Verification items for the finished model (mm, model axes). A direction names the side the tool comes from. Round coordinates to 2 decimals unless told otherwise and drop trailing zeros. Order: outer loops, then holes, each group sorted by start corner. A loop starts at its lowest first (then second) coordinate and runs counter-clockwise, first axis right, second up. Notation, with made-up numbers: (55, 10) -> (114, 10) arc R27 cw to (114, 29) -> close; hole circle Ø9 at (-27.75, -23). An arc over 180 degrees is marked (long way). Put each result on its own line as item: value.
from build123d import *
from build123d.topology import SkipClean

# Parameters (mm, degrees)
SKETCH1_R           = 21.082
SKETCH1_R_2         = 17.526
BOSS_EXTRUDE1_DEPTH = 254
BOSS_EXTRUDE2_START = 6.35
SKETCH2_R           = 21.082
BOSS_EXTRUDE2_DEPTH = 6.35
SKETCH3_R           = 25.868376463
CUT_EXTRUDE1_DEPTH  = 127
SKETCH4_R           = 34.925
SKETCH4_R_2         = 19.091061219
BOSS_EXTRUDE3_DEPTH = 3.175
CUT_EXTRUDE2_DEPTH  = 143.203142546
CIRPATTERN1_COUNT   = 12
SKETCH6_R           = 21.082
CUT_EXTRUDE3_DEPTH  = 6.35
SKETCH7_R           = 21.082
BOSS_EXTRUDE4_DEPTH = 6.35
CUT_EXTRUDE5_DEPTH  = 137.26632471
BOSS_EXTRUDE5_DEPTH = 3.175
SKETCH13_R          = 20.701
SKETCH13_R_2        = 18.0848
CUT_EXTRUDE6_DEPTH  = 1.016
SKETCH14_R          = 22.3012
SKETCH14_R_2        = 20.701
BOSS_EXTRUDE6_DEPTH = 3.175
SKETCH15_R          = 3.175
SKETCH15_R_2        = 21.082
BOSS_EXTRUDE7_DEPTH = 123.825
SKETCH17_R          = 47.464750001
SKETCH17_R_2        = 22.3012
CUT_EXTRUDE7_DEPTH  = 120.65
SKETCH18_R          = 17.526
CUT_EXTRUDE8_DEPTH  = 134.883658048
CUT_EXTRUDE9_START  = -1.016
SKETCH19_R          = 20.701
SKETCH19_R_2        = 18.0848
CUT_EXTRUDE9_DEPTH  = 1.016
SKETCH20_R          = 43.35542212
CUT_EXTRUDE10_DEPTH = 25.4
SKETCH21_R          = 25.927665562
CUT_EXTRUDE11_DEPTH = 38.1
SKETCH22_R          = 20.063036937
BOSS_EXTRUDE8_DEPTH = 3.175


with BuildPart() as part:
    # Sketch1 → Boss-Extrude1 (new body)
    with BuildSketch(Plane.XY):
        Circle(SKETCH1_R)
        Circle(SKETCH1_R_2, mode=Mode.SUBTRACT)
    extrude(amount=BOSS_EXTRUDE1_DEPTH)

    # Sketch2 → Boss-Extrude2 (add)
    with BuildSketch(Plane(origin=(0, 0, 0), x_dir=(-1, 0, 0), z_dir=(0, 0, -1)).offset(BOSS_EXTRUDE2_START)):
        Circle(SKETCH2_R)
    extrude(amount=-BOSS_EXTRUDE2_DEPTH)

    # Sketch3 → Cut-Extrude1 (cut)
    with BuildSketch(Plane.XY.offset(254)):
        Circle(SKETCH3_R)
    extrude(amount=-CUT_EXTRUDE1_DEPTH, mode=Mode.SUBTRACT)

    # Sketch4 → Boss-Extrude3 (add)
    with BuildSketch(Plane.XY.offset(127)):
        Circle(SKETCH4_R)
        Circle(SKETCH4_R_2, mode=Mode.SUBTRACT)
    extrude(amount=-BOSS_EXTRUDE3_DEPTH)

    # Sketch5 → Cut-Extrude2 (cut, through all)
    with BuildSketch(Plane.XY.offset(127)):
        with BuildLine():
            ThreePointArc((0, 31.75), (-3.175, 28.575), (0, 25.4))
            Line((0, 25.4), (0, 31.75))
        make_face()
        with BuildLine():
            Line((0, 31.75), (0, 25.4))
            ThreePointArc((0, 25.4), (2.24506403, 26.32993597), (3.175, 28.575))
            ThreePointArc((3.175, 28.575), (2.24506403, 30.82006403), (0, 31.75))
        make_face()
    cut_extrude2 = extrude(amount=-CUT_EXTRUDE2_DEPTH, mode=Mode.SUBTRACT)

    # CirPattern1: Cut-Extrude2 ×12 about axis
    cirpattern1_axis = Axis((0, 0, 0), (0, 0, 1))
    for i in range(1, CIRPATTERN1_COUNT):
        add(cut_extrude2.rotate(cirpattern1_axis, i * 360 / CIRPATTERN1_COUNT), mode=Mode.SUBTRACT)

    # Sketch6 → Cut-Extrude3 (cut)
    with BuildSketch(Plane(origin=(0, 0, -6.35), x_dir=(-1, 0, 0), z_dir=(0, 0, -1))):
        Circle(SKETCH6_R)
    extrude(amount=-CUT_EXTRUDE3_DEPTH, mode=Mode.SUBTRACT)

    # Sketch7 → Boss-Extrude4 (add)
    with BuildSketch(Plane(origin=(0, 0, 0), x_dir=(-1, 0, 0), z_dir=(0, 0, -1))):
        Circle(SKETCH7_R)
    extrude(amount=-BOSS_EXTRUDE4_DEPTH)

    # Sketch8 → Cut-Extrude5 (cut, through all)
    with BuildSketch(Plane.XY.offset(127)):
        with BuildLine():
            ThreePointArc((18.828599641, 18.828599641), (22.949516837, 21.527350272), (27.854121372, 21.069018667))
            ThreePointArc((27.854121372, 21.069018667), (0, 34.925), (-27.854121372, 21.069018667))
            ThreePointArc((-27.854121372, 21.069018667), (-22.949516837, 21.527350272), (-18.828599641, 18.828599641))
            Line((-18.828599641, 18.828599641), (-14.907225161, 14.907225161))
            ThreePointArc((-14.907225161, 14.907225161), (0, 21.082), (14.907225161, 14.907225161))
            Line((14.907225161, 14.907225161), (18.828599641, 18.828599641))
        make_face()
        with BuildLine():
            ThreePointArc((14.907225161, -14.907225161), (0, -21.082), (-14.907225161, -14.907225161))
            Line((-14.907225161, -14.907225161), (-18.828599641, -18.828599641))
            ThreePointArc((-18.828599641, -18.828599641), (-22.949516837, -21.527350272), (-27.854121372, -21.069018667))
            ThreePointArc((-27.854121372, -21.069018667), (0, -34.925), (27.854121372, -21.069018667))
            ThreePointArc((27.854121372, -21.069018667), (22.949516837, -21.527350272), (18.828599641, -18.828599641))
            Line((18.828599641, -18.828599641), (14.907225161, -14.907225161))
        make_face()
    extrude(amount=-CUT_EXTRUDE5_DEPTH, mode=Mode.SUBTRACT)

    # Sketch11 → Boss-Extrude5 (add)
    with BuildSketch(Plane.XY.offset(127)):
        with BuildLine():
            ThreePointArc((31.206854634, 18.017286001), (29.767943301, 19.804028486), (27.854121372, 21.069018667))
            ThreePointArc((27.854121372, 21.069018667), (34.925, 0), (27.854121372, -21.069018667))
            ThreePointArc((27.854121372, -21.069018667), (29.767943301, -19.804028486), (31.206854634, -18.017286001))
            ThreePointArc((31.206854634, -18.017286001), (36.034571885, 0), (31.206854634, 18.017286001))
        make_face()
        with BuildLine():
            ThreePointArc((-27.854121372, 21.069018667), (-29.767943301, 19.804028486), (-31.206854634, 18.017286001))
            ThreePointArc((-31.206854634, 18.017286001), (-36.034571885, -1.77e-07), (-31.206854456, -18.017286308))
            ThreePointArc((-31.206854456, -18.017286308), (-29.767943169, -19.804028605), (-27.854121372, -21.069018667))
            ThreePointArc((-27.854121372, -21.069018667), (-34.925, 0), (-27.854121372, 21.069018667))
        make_face()
    extrude(amount=-BOSS_EXTRUDE5_DEPTH)

    # Sketch13 → Cut-Extrude6 (cut)
    with BuildSketch(Plane.XY.offset(127)):
        Circle(SKETCH13_R)
        Circle(SKETCH13_R_2, mode=Mode.SUBTRACT)
    extrude(amount=-CUT_EXTRUDE6_DEPTH, mode=Mode.SUBTRACT)

    # Sketch14 → Boss-Extrude6 (add)
    with BuildSketch(Plane.XY.offset(127)):
        Circle(SKETCH14_R)
        Circle(SKETCH14_R_2, mode=Mode.SUBTRACT)
    extrude(amount=-BOSS_EXTRUDE6_DEPTH)

    # Sketch15 → Boss-Extrude7 (add)
    with BuildSketch(Plane(origin=(0, 0, 123.825), x_dir=(-1, 0, 0), z_dir=(0, 0, -1))):
        with BuildLine():
            ThreePointArc((31.206854667, 18.017285943), (25.234555257, 21.731100369), (18.828599641, 18.828599641))
            Line((18.828599641, 18.828599641), (15.769329749, 15.769329749))
            ThreePointArc((15.769329749, 15.769329749), (0, 22.3012), (-15.769329749, 15.769329749))
            Line((-15.769329749, 15.769329749), (-18.828599641, 18.828599641))
            ThreePointArc((-18.828599641, 18.828599641), (-25.234555257, 21.731100369), (-31.206854667, 18.017285943))
            ThreePointArc((-31.206854667, 18.017285943), (-36.034571885, 0), (-31.206854667, -18.017285943))
            ThreePointArc((-31.206854667, -18.017285943), (-25.234555257, -21.731100369), (-18.828599641, -18.828599641))
            Line((-18.828599641, -18.828599641), (-15.769329749, -15.769329749))
            ThreePointArc((-15.769329749, -15.769329749), (0, -22.3012), (15.769329749, -15.769329749))
            Line((15.769329749, -15.769329749), (18.828599641, -18.828599641))
            ThreePointArc((18.828599641, -18.828599641), (25.234555257, -21.731100369), (31.206854667, -18.017285943))
            ThreePointArc((31.206854667, -18.017285943), (36.034571885, 0), (31.206854667, 18.017285943))
        make_face()
        with Locations(Location((28.575, 0, 0), (0, 0, 90))):
            Circle(SKETCH15_R, mode=Mode.SUBTRACT)
        with Locations(Location((-24.746675913, -14.2875, 0), (0, 0, 300))):
            Circle(SKETCH15_R, mode=Mode.SUBTRACT)
        with Locations(Location((-24.746675913, 14.2875, 0), (0, 0, 240))):
            Circle(SKETCH15_R, mode=Mode.SUBTRACT)
        with Locations(Location((-28.575, 0, 0), (0, 0, 270))):
            Circle(SKETCH15_R, mode=Mode.SUBTRACT)
        Circle(SKETCH15_R_2, mode=Mode.SUBTRACT)
        with Locations(Location((24.746675913, -14.2875, 0), (0, 0, 60))):
            Circle(SKETCH15_R, mode=Mode.SUBTRACT)
        with Locations(Location((24.746675913, 14.2875, 0), (0, 0, 120))):
            Circle(SKETCH15_R, mode=Mode.SUBTRACT)
    extrude(amount=BOSS_EXTRUDE7_DEPTH)

    # Sketch17 → Cut-Extrude7 (cut)
    with BuildSketch(Plane.XY.offset(123.825)):
        Circle(SKETCH17_R)
        with Locations(Location((0, 0, 0), (0, 0, 315))):
            Circle(SKETCH17_R_2, mode=Mode.SUBTRACT)
    extrude(amount=-CUT_EXTRUDE7_DEPTH, mode=Mode.SUBTRACT)

    # Sketch18 → Cut-Extrude8 (cut, through all)
    with BuildSketch(Plane.XY.offset(127)):
        Circle(SKETCH18_R)
    extrude(amount=-CUT_EXTRUDE8_DEPTH, mode=Mode.SUBTRACT)

    # Sketch19 → Cut-Extrude9 (cut)
    with BuildSketch(Plane(origin=(0, 0, 0), x_dir=(-1, 0, 0), z_dir=(0, 0, -1)).offset(CUT_EXTRUDE9_START)):
        with Locations(Location((0, 0, 0), (0, 0, 180))):
            Circle(SKETCH19_R)
        with Locations(Location((0, 0, 0), (0, 0, 180))):
            Circle(SKETCH19_R_2, mode=Mode.SUBTRACT)
    extrude(amount=CUT_EXTRUDE9_DEPTH, mode=Mode.SUBTRACT)

    # Sketch20 → Cut-Extrude10 (cut)
    with SkipClean():  # the faces are left unmerged after this step: merging them gives an invalid solid
        with BuildSketch(Plane(origin=(0, 0, 0), x_dir=(-1, 0, 0), z_dir=(0, 0, -1))):
            Circle(SKETCH20_R)
        extrude(amount=-CUT_EXTRUDE10_DEPTH, mode=Mode.SUBTRACT)

    # Sketch21 → Cut-Extrude11 (cut)
    with SkipClean():  # the faces are left unmerged after this step: merging them gives an invalid solid
        with BuildSketch(Plane(origin=(0, 0, 25.4), x_dir=(-1, 0, 0), z_dir=(0, 0, -1))):
            Circle(SKETCH21_R)
        extrude(amount=-CUT_EXTRUDE11_DEPTH, mode=Mode.SUBTRACT)

    # Sketch22 → Boss-Extrude8 (add)
    with SkipClean():  # the faces are left unmerged after this step: merging them gives an invalid solid
        with BuildSketch(Plane(origin=(0, 0, 63.5), x_dir=(-1, 0, 0), z_dir=(0, 0, -1))):
            Circle(SKETCH22_R)
        extrude(amount=-BOSS_EXTRUDE8_DEPTH)


solid = part.part
Item 1: Gauge pin test, flat ends, axial feed: pin 1 Ø10.5 at (x, y) = (2, 3.5) entering from +Z (3 decimals); pin 2 Ø22.5 at (x, y) = (-26.5, 3.5) entering from -Z; pin 3 Ø12 at (y, z) = (-13.5, 91.5) entering from +X; pin 4 Ø12 at (y, z) = (4.5, 112) entering from -X. Record the tip position at first contact, or that the pin passes through.
Check sheet entries:
pin 1: stops at z = 66.675
pin 2: stops at z = 63.5
pin 3: stops at x = 21
pin 4: stops at x = -22.3
Item 2: Material ranges on L1, parallel to Y at x = 0, z = 126.75; L2, parallel to Y at x = 0, z = 100, recorded low to high. Write a range as [from, to].
Check sheet entries:
L1: y = [-22.3, -20.7], [-18.08, -17.53], [17.53, 18.08], [20.7, 22.3]
L2: y = [-22.3, -17.53], [17.53, 22.3]
Item 3: Release check for a two-part mould opening along X. For faces 1 (the flat face through (0, 0, 63.5)), 2 (the cylindrical face through (-36.034, 0.264, 125.435)), 3 (the flat face through (-17, -17, 125)) record: +X half, -X half, draft (parallel to the pull), parting line (faces both ways), or undercut.
Check sheet entries:
face 1: draft
face 2: -X half
face 3: undercut
Item 4: Section check B-B on x = 0. Record the boundary of the cut face in (y, z) (3 decimals).
Check sheet entries:
outline: (-22.301, 63.5) -> (22.301, 63.5) -> (22.301, 127) -> (20.701, 127) -> (20.701, 125.984) -> (18.085, 125.984) -> (18.085, 127) -> (17.526, 127) -> (17.526, 66.675) -> (-17.526, 66.675) -> (-17.526, 127) -> (-18.085, 127) -> (-18.085, 125.984) -> (-20.701, 125.984) -> (-20.701, 127) -> (-22.301, 127) -> close
Item 5: Section check A-A on z = 77.5. Record the boundary of the cut face in (x, y).
Check sheet entries:
outline: circle Ø44.6 at (0, 0); hole circle Ø35.05 at (0, 0)
Item 6: Tool access check on faces 4 (the flat face through (-17, 17, 125)), 5 (the flat face through (-2.8, 17.5, 127)), 6 (the cylindrical face through (36.034, 0.264, 125.435)), 7 (the flat face through (17, -17, 125)), 8 (the cylindrical face through (-16.428, -12.596, 126.499)). Record the directions out of +Z, -Z, +X, -X, +Y, -Y that give a thin tool (end or side, any length) a straight path to the whole face; none if there is none.
Check sheet entries:
face 4: +Z, -Z, +Y
face 5: +Z, +X, -X, +Y, -Y
face 6: +Z, -Z, +X
face 7: +Z, -Z, -Y
face 8: +Z
Item 7: Section check C-C on y = 4.5. Record the boundary of the cut face in (x, z) (3 decimals), then the cut area to 3 significant figures.
Check sheet entries:
outline: (-35.752, 123.825) -> (-21.842, 123.825) -> (-21.842, 63.5) -> (21.842, 63.5) -> (21.842, 123.825) -> (35.752, 123.825) -> (35.752, 127) -> (20.206, 127) -> (20.206, 125.984) -> (17.516, 125.984) -> (17.516, 127) -> (16.938, 127) -> (16.938, 66.675) -> (-16.938, 66.675) -> (-16.938, 127) -> (-17.516, 127) -> (-17.516, 125.984) -> (-20.206, 125.984) -> (-20.206, 127) -> (-35.752, 127) -> close
area: 813 mm^2
Item 8: Section check D-D on y = -9.5. Record the boundary of the cut face in (x, z) (3 decimals).
Check sheet entries:
outline: (-34.76, 123.825) -> (-20.177, 123.825) -> (-20.177, 63.5) -> (20.177, 63.5) -> (20.177, 123.825) -> (34.76, 123.825) -> (34.76, 127) -> (18.392, 127) -> (18.392, 125.984) -> (15.389, 125.984) -> (15.389, 127) -> (14.728, 127) -> (14.728, 66.675) -> (-14.728, 66.675) -> (-14.728, 127) -> (-15.389, 127) -> (-15.389, 125.984) -> (-18.392, 125.984) -> (-18.392, 127) -> (-34.76, 127) -> close
